Source: CAD feature listing. Evaluate the final solid. Frame: model axes, mm. Face numbers are marked on the shaded views. A direction names the side the tool comes from. Give positions to 0.01 mm unless a question says otherwise; leave off trailing zeros. Order: outer loops, then holes, each group sorted by start corner. A loop starts at its lowest first (then second) coordinate and runs counter-clockwise, first axis right, second up.
1) Access query for the marked faces 4 and 5. Directions: +Z, -Z, +X, -X, +Y, -Y. A direction counts if a zero-diameter tool reaches every point of the face in a straight line with its end or side. Return the directions, or none.
2) Draft query along Z for the marked faces 1, 2 and 3. Return one class per face: released by +Z, released by -Z, zero draft, split by the parting line, or undercut.
3) Section C-C, the plane x = 14. Return loops of the section in (y, z), plus the area to 3 significant figures.
4) Section B-B, the plane y = 0. Return loops of the section in (x, z).
5) Material intervals for line 1 (Y direction, x = 25.85, z = 0); line 2 (Y direction, x = 7.75, z = -1); line 3 (X direction, y = 22.2, z = 0), sorted ascending.
6) Section D-D, the plane y = 33.5. Return loops of the section in (x, z), plus the area to 3 significant figures.
7) First-contact query: P1, Ø6, axis at y = 5, z = 16.5, coming from the +X side; P2, Ø10, axis at x = 8.5, z = 16.5, coming from the +Y side; P3, Ø12.5, axis at y = 8, z = -8.5, coming from the -X side; P4, Ø9, axis at y = 24.75, z = 24.75, coming from the +X side. Flat tips, straight axial feed; report the tip coordinate or a pass-through.
8) Section A-A, the plane z = 0. Give the number of separate pieces and of enclosed holes in the cut face, plus the area to 3 significant figures.
```python
from build123d import *

# Parameters (mm, degrees)
HOLE_WIZARD_M8_1_D           = 6.8
HOLE_WIZARD_M8_1_CSINK_D     = 8.05
HOLE_WIZARD_M8_1_CSINK_ANGLE = 90
PATTERN_CIRCULAR_1_COUNT     = 4


# Read off the part's stored shape, not the designer's step: Ø3.0mm 暗销孔1
with BuildPart() as part:
    # 草图1 → 旋转1 (revolve)
    with BuildSketch(Plane.XY, mode=Mode.PRIVATE) as revolve_1_sk:
        Polygon((0, 0), (0, 42.5), (8, 42.5), (8, 25), (28, 25), (28, 0), align=None)
    revolve(revolve_1_sk.sketch.rotate(Axis((0, 0, 0), (1, 0, 0)), 90), axis=Axis((0, 0, 0), (1, 0, 0)))

    # 草图2 → 切除-旋转1 (revolve, cut)
    with BuildSketch(Plane.XY, mode=Mode.PRIVATE) as cut_revolve_1_sk:
        with BuildLine():
            Line((0, 0), (0, 20))
            Line((0, 20), (4, 20))
            Line((4, 20), (4, 21))
            ThreePointArc((4, 21), (5, 22), (6, 21))
            Line((6, 21), (22, 21))
            ThreePointArc((22, 21), (23, 22), (24, 21))
            Line((24, 21), (24, 20))
            Line((24, 20), (28, 20))
            Line((28, 20), (28, 0))
            Line((28, 0), (0, 0))
        make_face()
    revolve(cut_revolve_1_sk.sketch.rotate(Axis((0, 0, 0), (1, 0, 0)), 90), axis=Axis((0, 0, 0), (1, 0, 0)), mode=Mode.SUBTRACT)

    # Ø3.0mm 暗销孔1 outline → Ø3.0mm 暗销孔1 (revolve, cut)
    with BuildSketch(Plane(origin=(18, 0, 0), x_dir=(1, 0, 0), z_dir=(0, 0, 1))):
        Polygon((3.000038896, 25.000038896), (0, 25.000038896), (0, 20.946331159), (1.5, 20.946331159), (1.5, 23.5), align=None)
    revolve(axis=Axis((18, 0, 0), (0, 1, 0)), mode=Mode.SUBTRACT)

    # M8 螺纹孔1 (through all)
    with Locations(Plane.ZY):
        with Locations((24.748737342, 24.748737342)):
            hole_wizard_m8_1 = CounterSinkHole(HOLE_WIZARD_M8_1_D / 2, HOLE_WIZARD_M8_1_CSINK_D / 2, counter_sink_angle=HOLE_WIZARD_M8_1_CSINK_ANGLE)

    # 阵列(圆周)1: M8 螺纹孔1 ×4 about axis
    pattern_circular_1_axis = Axis((0, 0, 0), (1, 0, 0))
    for i in range(1, PATTERN_CIRCULAR_1_COUNT):
        add(hole_wizard_m8_1.rotate(pattern_circular_1_axis, i * 360 / PATTERN_CIRCULAR_1_COUNT), mode=Mode.SUBTRACT)


solid = part.part
```
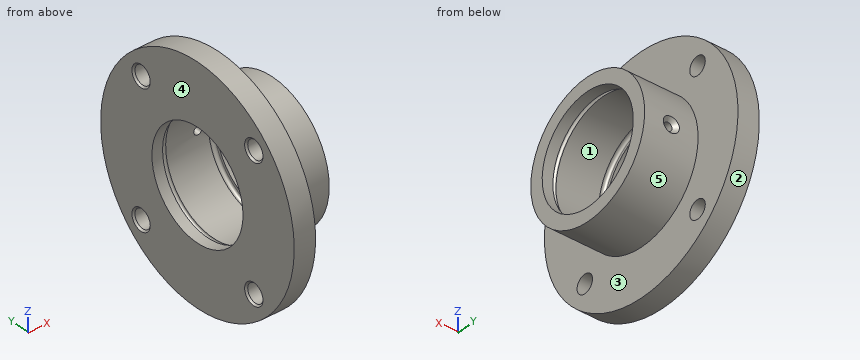
From the geometry:
1. face 4: +Z, -Z, -X, +Y, -Y
1. face 5: +X
2. face 1: undercut
2. face 2: split by the parting line
2. face 3: zero draft
3. outline: circle Ø50 at (0, 0); hole circle Ø42 at (0, 0)
3. area: 578 mm2
4. outline: (0, -42.5) - (8, -42.5) - (8, -25) - (28, -25) - (28, -20) - (24, -20) - (24, -21) arc R1 cw to (22, -21) - (6, -21) arc R1 cw to (4, -21) - (4, -20) - (0, -20) - close; (0, 20) - (4, 20) - (4, 21) arc R1 cw to (6, 21) - (22, 21) arc R1 cw to (24, 21) - (24, 20) - (28, 20) - (28, 25) - (8, 25) - (8, 42.5) - (0, 42.5) - close
5. line 1: y = -25 to -20, 20 to 25
5. line 2: y = -42.49 to -20.98, 20.98 to 42.49
5. line 3: x = 0 to 16.5, 19.5 to 28
6. outline: (0, -26.15) - (8, -26.15) - (8, 26.15) - (0, 26.15) - close
6. area: 418 mm2
7. P1: stops at x = 28
7. P2: stops at y = 40.91
7. P3: passes through
7. P4: stops at x = 8
8. separate pieces: 3
8. enclosed holes: 0
8. area: 499 mm2
